Source: CAD feature listing. Evaluate the final solid. Frame: model axes, mm. Face numbers are marked on the shaded views. Give positions to 0.01 mm unless a question says otherwise; leave off trailing zeros. Order: outer loops, then holes, each group sorted by start corner. A loop starts at its lowest first (then second) coordinate and runs counter-clockwise, first axis right, second up. Notation, with made-up numbers: M 42.25,73.5 L 57.25,73.5 A16 cw 57.25,90.5 Z; hole C 31,84 d2. An arc over 180 degrees is marked long. Use CSV: the item, a comma, the result in double quotes. Start each with the question number.
Item 1: Pull-direction query (Z, two-part tool) for the marked faces 1 and 2; classes: +Z half, -Z half, draft (parallel to the pull), parting line (faces both ways), or undercut.
Item 2: First-contact query: pin 1 (2 mm diameter, centred on y = 5, z = -6, fed in from +X); pin 2 (3 mm diameter, centred on x = 3.5, y = 4, fed in from +Z); pin 3 (1 mm diameter, centred on y = 4.5, z = 7, fed in from -X). Flat tips, straight axial feed; report the tip coordinate or a pass-through.
Item 3: Ray query, probe 1 along Y at (x, z) = (-5, 7); probe 2 along X at (y, z) = (3.8, 0); probe 3 along X at (y, z) = (3.1, 0). Return the intervals inside material, ascending. Write a range as from..to.
Item 4: Section query D-D on z = -8.5. Return loops of the section in (x, y).
Item 5: Section query C-C on y = 0.85. Return loops of the section in (x, z), and give its area (3 significant figures).
Autodesk Inventor part; units mm, degrees
ref_plane "YZ Plane" through (0, 0, 0) normal (1, 0, 0) x (0, 1, 0)
ref_plane "XZ Plane" through (0, 0, 0) normal (0, 1, 0) x (-1, 0, 0)
ref_plane "XY Plane" through (0, 0, 0) normal (0, 0, 1) x (1, 0, 0)
sketch "Sketch1" plane through (0, 0, 0) normal (0, 1, 0) x (-1, 0, 0)
  circle A0 centre (0, 0) radius 9.5
  dimension "d0" = 19
extrude "Extrusion1" add sketch "Sketch1" along normal blind 1.25
sketch "Sketch2" plane through (0, 1.25, 0) normal (0, 1, 0) x (1, 0, 0)
  circle A0 centre (0, 0) radius 8
  dimension "d3" = 16
extrude "Extrusion2" add sketch "Sketch2" along normal blind 0.5
sketch "Sketch3" plane through (0, 1.75, 0) normal (0, 1, 0) x (1, 0, 0)
  circle A0 centre (0, 0) radius 9.5
  dimension "d6" = 19
extrude "Extrusion3" add sketch "Sketch3" along normal blind 1
sketch "Sketch4" plane through (0, 2.75, 0) normal (0, 1, 0) x (1, 0, 0)
  circle A0 centre (0, 0) radius 8
  dimension "d9" = 16
extrude "Extrusion4" add sketch "Sketch4" along normal blind 0.5
sketch "Sketch5" plane through (0, 3.25, 0) normal (0, 1, 0) x (1, 0, 0)
  circle A0 centre (0, 0) radius 9.5
  dimension "d12" = 19
extrude "Extrusion5" add sketch "Sketch5" along normal blind 1
sketch "Sketch6" plane through (0, 4.25, 0) normal (0, 1, 0) x (1, 0, 0)
  circle A0 centre (0, 0) radius 42.9812
  circle A1 centre (0, 0) radius 8
  dimension "d15" = 16
extrude "Extrusion6" add sketch "Sketch6" along normal blind 0.5 contours A1
sketch "Sketch7" plane through (0, 4.75, 0) normal (0, 1, 0) x (1, 0, 0)
  circle A0 centre (0, 0) radius 9.5
  dimension "d18" = 19
extrude "Extrusion7" add sketch "Sketch7" along normal blind 1.25
sketch "Sketch8" plane through (0, 6, 0) normal (0, 1, 0) x (1, 0, 0)
  circle A0 centre (0, 0) radius 1.5
  dimension "d21" = 3
hole "Hole1" at (0, 6, 0) direction (0, -1, 0) diameter 3 end through all
thread "Thread1"
properties material "Brass, Soft Yellow, Welded"
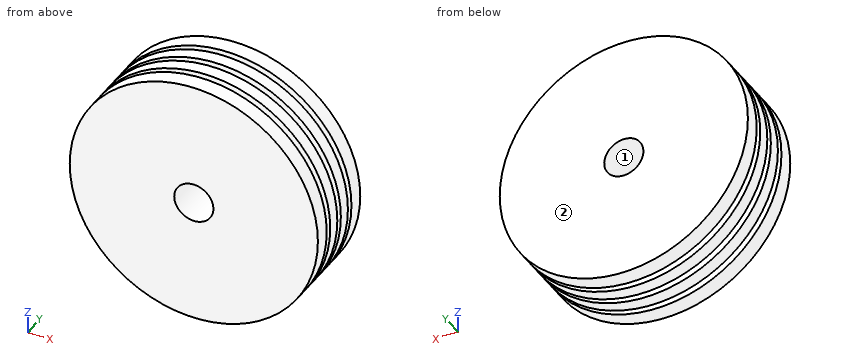
Verdict:
1,face 1,"undercut"
1,face 2,"draft"
2,pin 1,"x = 8.08"
2,pin 2,"z = 9.29"
2,pin 3,"x = -6.86"
3,probe 1,"0..1.25, 1.75..2.75, 3.25..4.25, 4.75..6"
3,probe 2,"-9.5..-1.5, 1.5..9.5"
3,probe 3,"-8..-1.5, 1.5..8"
4,outline,"M -4.24,0 L 4.24,0 L 4.24,1.25 L -4.24,1.25 Z; M -4.24,1.75 L 4.24,1.75 L 4.24,2.75 L -4.24,2.75 Z; M -4.24,3.25 L 4.24,3.25 L 4.24,4.25 L -4.24,4.25 Z; M -4.24,4.75 L 4.24,4.75 L 4.24,6 L -4.24,6 Z"
5,outline,"C 0,0 d19; hole C 0,0 d3"
5,area,"276 mm2"
